```python
from build123d import *

# Parameters (mm, degrees)
SKETCH3_W           = 32.004
SKETCH3_H           = 38.1
BOSS_EXTRUDE1_DEPTH = 3.175
SKETCH4_R           = 2.54
SCREW_HOLES_DEPTH   = 26.080811969
SKETCH5_W           = 16.51
SKETCH5_H           = 25.4
WHEEL_APPROX_DEPTH  = 32.004


with BuildPart() as part:
    # Sketch3 → Boss-Extrude1 (new body)
    with BuildSketch(Plane(origin=(0, 0, 0), x_dir=(1, 0, 0), z_dir=(0, 1, 0))):
        Rectangle(SKETCH3_W, SKETCH3_H)
    extrude(amount=-BOSS_EXTRUDE1_DEPTH)

    # Sketch4 → Screw Holes (cut, through all)
    with BuildSketch(Plane(origin=(0, 0, 0), x_dir=(1, 0, 0), z_dir=(0, 1, 0))):
        with Locations(Location((11.938, 15.24, 0), (0, 0, 270))):
            Circle(SKETCH4_R)
        with Locations(Location((-11.938, 15.24, 0), (0, 0, 270))):
            Circle(SKETCH4_R)
        with Locations(Location((-11.938, -15.24, 0), (0, 0, 270))):
            Circle(SKETCH4_R)
        with Locations(Location((11.938, -15.24, 0), (0, 0, 270))):
            Circle(SKETCH4_R)
    extrude(amount=-SCREW_HOLES_DEPTH, mode=Mode.SUBTRACT)

    # Sketch5 → Wheel Approx (add)
    with BuildSketch(Plane(origin=(0, 0, 0), x_dir=(1, 0, 0), z_dir=(0, 1, 0))):
        Rectangle(SKETCH5_W, SKETCH5_H)
    extrude(amount=-WHEEL_APPROX_DEPTH)


solid = part.part
```
CAD build for the part. Positions are in the model's coordinates, mm. A direction names the side the tool comes from. Coordinates: 2 decimals unless noted, no trailing zeros. Order: outer loops, then holes, each group sorted by start corner. A loop starts at its lowest first (then second) coordinate and runs counter-clockwise, first axis right, second up. Notation, with made-up numbers: M -18,79 L 27,79 A14 ccw 27,89 Z; hole C 89.25,10.5 d10. An arc over 180 degrees is marked long. Write each question's results on one line, items separated by ' | '. Start each with the question number.
Q1. Cut at D-D (y = -26). List the corners of the cut face in (x, z) (3 decimals), then the cut area to 3 significant figures.
Q2. Drill centre lines: probe 1 along X at (y, z) = (-1, 15); probe 2 along Z at (x, y) = (2.5, -8); probe 3 along X at (y, z) = (-22, -12) (3 decimals). Where is each one in solid material? Low to high. Write a range as from..to.
Q3. Pull direction Z, two halves, no side cores. Call faces 6 (the flat face through (0, -2, -19.05)), 7 (the flat face through (16.002, -2, 0)), 8 (the cylindrical face through (-9.8, -1.57, -13.87)): +Z half, -Z half, draft (parallel to the pull), parting line (faces both ways), or undercut.
Q4. Cut at C-C (z = -8). List the corners of the cut face in (x, y) (3 decimals), then the cut area to 3 significant figures.
Q5. Flat gauge pins, fed straight in: P1, Ø6, axis at x = 11.938, z = -15.24, coming from the +Y side; P2, Ø8, axis at x = 4.5, y = -25.5, coming from the +Z side; P3, Ø12, axis at y = -23, z = -14.5, coming from the -X side (3 decimals); P4, Ø8.5, axis at x = -1, y = -17.5, coming from the -Z side. Where does each tip first touch, or does it go through?
Q6. Cut at B-B (x = 2.5). List the corners of the cut face in (y, z) (3 decimals), then the cut area to 3 significant figures.
Q7. Which spindle directions (+Z, -Z, +X, -X, +Y, -Y) get a long thin tool onto all of the face, cutting with end or side? Do faces 1 (the flat face through (8.255, -17, 0)), 2 (the flat face through (0, -17, -12.7)), 3 (the flat face through (-8.255, -17, 0)), 4 (the flat face through (0, 0, 0)), 5 (the flat face through (0, -17, 12.7)). Say none if no direction does.
Q8. Cut at A-A (z = -15.24). List the corners of the cut face in (x, y) (3 decimals).
Found:
1) outline: M -8.255,-12.7 L 8.255,-12.7 L 8.255,12.7 L -8.255,12.7 Z | area: 419 mm²
2) probe 1: -16..-14.47, -9.41..9.41, 14.47..16 | probe 2: -12.7..12.7 | probe 3: -8.255..8.255
3) face 6: -Z half | face 7: draft | face 8: undercut
4) outline: M -16.002,-3.175 L -8.255,-3.175 L -8.255,-32.004 L 8.255,-32.004 L 8.255,-3.175 L 16.002,-3.175 L 16.002,0 L -16.002,0 Z | area: 578 mm²
5) P1: y = 0 | P2: z = 12.7 | P3: x = -8.255 | P4: z = -12.7
6) outline: M -32.004,-12.7 L -3.175,-12.7 L -3.175,-19.05 L 0,-19.05 L 0,19.05 L -3.175,19.05 L -3.175,12.7 L -32.004,12.7 Z | area: 853 mm²
7) face 1: +Z, -Z, +X, -Y | face 2: -Z, +X, -X, -Y | face 3: +Z, -Z, -X, -Y | face 4: +Z, -Z, +X, -X, +Y | face 5: +Z, +X, -X, -Y
8) outline: M -16.002,-3.175 L -14.478,-3.175 L -14.478,0 L -16.002,0 Z; M -9.398,-3.175 L 9.398,-3.175 L 9.398,0 L -9.398,0 Z; M 14.478,-3.175 L 16.002,-3.175 L 16.002,0 L 14.478,0 Z
